Part print with two shaded views. Sizes in mm from the minimum x, y, z corner. Round coordinates to 2 decimals unless told otherwise and drop trailing zeros. Write each loop counter-clockwise with the first axis right and the second up, starting at its lowest first coordinate (ties: lowest second). Pieces come first, ordered by that corner, then holes. Notation, with made-up numbers: (55.25, 48) -> (77.25, 48) arc R34 cw to (77.25, 80) -> close; hole circle Ø6 at (-20, -26). An arc over 180 degrees is marked (long way). Answer in a Markdown table with one row per item.
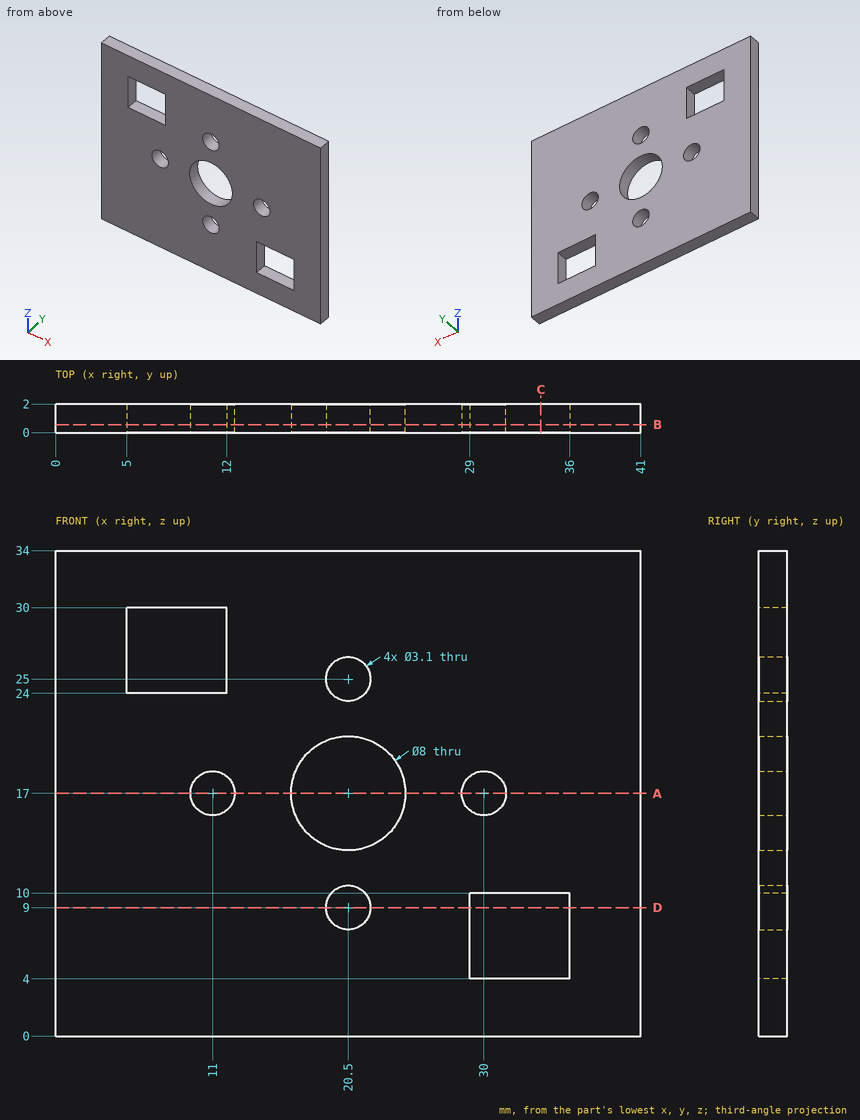
Q1. Saw through at B-B on y = 0.55. Write the cut outline in (x, z), plus the area to 3 significant figures.
A:
| item | result |
|---|---|
| outline | (0, 0) -> (41, 0) -> (41, 34) -> (0, 34) -> close; hole (5, 24) -> (12, 24) -> (12, 30) -> (5, 30) -> close; hole circle Ø3.1 at (11, 17); hole circle Ø8 at (20.5, 17); hole circle Ø3.1 at (20.5, 9); hole circle Ø3.1 at (20.5, 25); hole circle Ø3.1 at (30, 17); hole (29, 4) -> (36, 4) -> (36, 10) -> (29, 10) -> close |
| area | 1,230 mm² |
Q2. Wall check: line 1 (Z direction, x = 20.5, y = 0.8); line 2 (Z direction, x = 30, y = 1.2); line 3 (X direction, y = 1.85, z = 29). Give the ranges that are in metal, low to high. Write a range as [from, to].
A:
| item | result |
|---|---|
| line 1 | [0, 7.45], [10.55, 13], [21, 23.45], [26.55, 34] |
| line 2 | [0, 4], [10, 15.45], [18.55, 34] |
| line 3 | [0, 5], [12, 41] |
Q3. Saw through at C-C on x = 34. Write the cut outline in (y, z), plus the area to 3 significant figures.
A:
| item | result |
|---|---|
| outline | (0, 0) -> (2, 0) -> (2, 4) -> (0, 4) -> close; (0, 10) -> (2, 10) -> (2, 34) -> (0, 34) -> close |
| area | 56.0 mm² |
Q4. Saw through at D-D on z = 9. Write the cut outline in (x, y), plus the area to 3 significant figures.
A:
| item | result |
|---|---|
| outline | (0, 0) -> (18.95, 0) -> (18.95, 2) -> (0, 2) -> close; (22.05, 0) -> (29, 0) -> (29, 2) -> (22.05, 2) -> close; (36, 0) -> (41, 0) -> (41, 2) -> (36, 2) -> close |
| area | 61.8 mm² |
Q5. Saw through at A-A on z = 17. Write the cut outline in (x, y).
A:
| item | result |
|---|---|
| outline | (0, 0) -> (9.45, 0) -> (9.45, 2) -> (0, 2) -> close; (12.55, 0) -> (16.5, 0) -> (16.5, 2) -> (12.55, 2) -> close; (24.5, 0) -> (28.45, 0) -> (28.45, 2) -> (24.5, 2) -> close; (31.55, 0) -> (41, 0) -> (41, 2) -> (31.55, 2) -> close |
